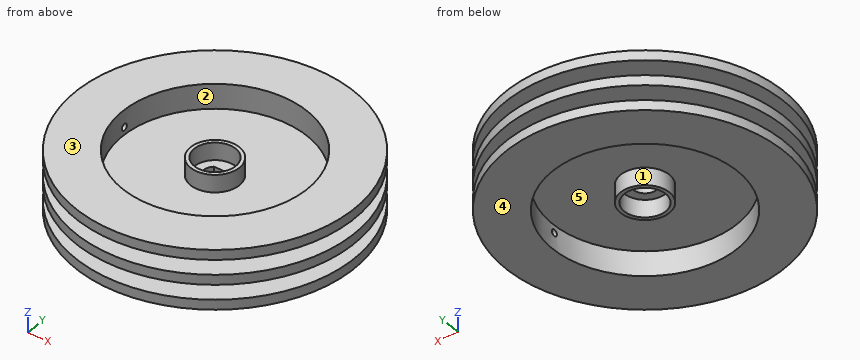
```python
from build123d import *

# Parameters (mm, degrees)
SKETCH1_R               = 23.9268
BOSS_EXTRUDE1_DEPTH     = 1.70942
SKETCH2_R               = 19.0119
BOSS_EXTRUDE2_DEPTH     = 2.54
SKETCH3_R               = 19.0119
BOSS_EXTRUDE3_DEPTH     = 2.54
SKETCH4_R               = 23.9268
BOSS_EXTRUDE4_DEPTH     = 1.70942
SKETCH5_R               = 23.9268
BOSS_EXTRUDE5_DEPTH     = 1.70942
SKETCH6_R               = 15.875
CUT_EXTRUDE1_DEPTH      = 4.24942
SKETCH7_R               = 15.875
CUT_EXTRUDE2_DEPTH      = 4.24942
SKETCH8_R               = 0.5715
CUT_EXTRUDE3_DEPTH      = 24.9268
CUT_EXTRUDE3_DEPTH_BACK = 24.9268
CUT_EXTRUDE4_DEPTH      = 6.9588401
SKETCH10_R              = 4.1975
SKETCH10_R_2            = 3.5625
BOSS_EXTRUDE7_DEPTH     = 3
SKETCH11_R              = 4.1975
SKETCH11_R_2            = 3.5625
BOSS_EXTRUDE8_DEPTH     = 3


with BuildPart() as part:
    # Sketch1 → Boss-Extrude1 (new body)
    with BuildSketch(Plane.XY):
        Circle(SKETCH1_R)
    extrude(amount=BOSS_EXTRUDE1_DEPTH)

    # Sketch2 → Boss-Extrude2 (add)
    with BuildSketch(Plane.XY.offset(1.70942)):
        Circle(SKETCH2_R)
    extrude(amount=BOSS_EXTRUDE2_DEPTH)

    # Sketch3 → Boss-Extrude3 (add)
    with BuildSketch(Plane(origin=(0, 0, 0), x_dir=(-1, 0, 0), z_dir=(0, 0, -1))):
        Circle(SKETCH3_R)
    extrude(amount=BOSS_EXTRUDE3_DEPTH)

    # Sketch4 → Boss-Extrude4 (add)
    with BuildSketch(Plane.XY.offset(4.24942)):
        Circle(SKETCH4_R)
    extrude(amount=BOSS_EXTRUDE4_DEPTH)

    # Sketch5 → Boss-Extrude5 (add)
    with BuildSketch(Plane(origin=(0, 0, -2.54), x_dir=(-1, 0, 0), z_dir=(0, 0, -1))):
        Circle(SKETCH5_R)
    extrude(amount=BOSS_EXTRUDE5_DEPTH)

    # Sketch6 → Cut-Extrude1 (cut)
    with BuildSketch(Plane.XY.offset(5.95884)):
        Circle(SKETCH6_R)
    extrude(amount=-CUT_EXTRUDE1_DEPTH, mode=Mode.SUBTRACT)

    # Sketch7 → Cut-Extrude2 (cut)
    with BuildSketch(Plane(origin=(0, 0, -4.24942), x_dir=(-1, 0, 0), z_dir=(0, 0, -1))):
        Circle(SKETCH7_R)
    extrude(amount=-CUT_EXTRUDE2_DEPTH, mode=Mode.SUBTRACT)

    # Sketch8 → Cut-Extrude3 (cut, two sides)
    with BuildSketch(Plane(origin=(0, 0, 0), x_dir=(0, 0, -1), z_dir=(1, 0, 0))) as cut_extrude3_sk:
        with Locations((-2.97942, 0)):
            Circle(SKETCH8_R)
        with Locations((1.27, 0)):
            Circle(SKETCH8_R)
    extrude(amount=CUT_EXTRUDE3_DEPTH, mode=Mode.SUBTRACT)
    extrude(cut_extrude3_sk.sketch, amount=-CUT_EXTRUDE3_DEPTH_BACK, mode=Mode.SUBTRACT)

    # Sketch9 → Cut-Extrude4 (cut, through all)
    with BuildSketch(Plane.XY.offset(1.70942)):
        with BuildLine():
            Line((-1.322875656, 1.5), (1.322875656, 1.5))
            ThreePointArc((1.322875656, 1.5), (0, -2), (-1.322875656, 1.5))
        make_face()
    extrude(amount=-CUT_EXTRUDE4_DEPTH, mode=Mode.SUBTRACT)

    # Sketch10 → Boss-Extrude7 (add)
    with BuildSketch(Plane.XY.offset(1.70942)):
        Circle(SKETCH10_R)
        Circle(SKETCH10_R_2, mode=Mode.SUBTRACT)
    extrude(amount=BOSS_EXTRUDE7_DEPTH)

    # Sketch11 → Boss-Extrude8 (add)
    with BuildSketch(Plane(origin=(0, 0, 0), x_dir=(-1, 0, 0), z_dir=(0, 0, -1))):
        Circle(SKETCH11_R)
        Circle(SKETCH11_R_2, mode=Mode.SUBTRACT)
    extrude(amount=BOSS_EXTRUDE8_DEPTH)


solid = part.part
```
Here's how the part is built. I have some questions about the finished solid (model axes, mm). Face numbers are marked on the shaded views. A direction names the side the tool comes from. Coordinates: 2 decimals unless noted, no trailing zeros. Order: outer loops, then holes, each group sorted by start corner. A loop starts at its lowest first (then second) coordinate and runs counter-clockwise, first axis right, second up. Notation, with made-up numbers: (25.5, 50.5) - (60.5, 50.5) arc R19 ccw to (60.5, 71.5) - close; hole circle Ø3 at (18, -39.5). An arc over 180 degrees is marked (long way). One line per question, with ' | ' between items. Start each with the question number.
1. If we section it at A-A (z = -1.27): Give the number of separate pieces and of enclosed holes in the cut face, and give its area (3 significant figures).
2. I'm going to push flat-ended pins straight in: pin 1 Ø6 at (y, z) = (17.5, -3) entering from -X; pin 2 Ø4.5 at (x, y) = (0, 0) entering from -Z; pin 3 Ø6 at (x, z) = (-2, 3) entering from -Y. Where does each tip first touch, or does it pass through?
3. If we section it at B-B (x = 17): Write out the boundary of the cut face in (y, z).
4. If we section it at D-D (x = -6): Write out the boundary of the cut face in (y, z).
5. Please list where these lines run through material, in increasing order: line 1 along Z through (x, y) = (21, 3.5); line 2 along Y through (x, z) = (0, -2.45) (1 decimal); line 3 along X through (y, z) = (2, 3). Write a range as [from, to].
6. Which directions (+Z, -Z, +X, -X, +Y, -Y) give clear straight access to the entire face, cutting with the end or side of a thin tool? Please do the marked faces 1, 2 and 3.
7. If we mould it in two halves opening along X, with no side actions, what happens to the marked faces 4 and 5? For each: released by +X, released by -X, zero draft, split by the parting line, or undercut.
8. If we section it at C-C (y = -17): Write out the boundary of the cut face in (x, z), and give its area (3 significant figures).
Model answer:
1) separate pieces: 3 | enclosed holes: 1 | area: 352 mm²
2) pin 1: stops at x = -19.03 | pin 2: stops at z = 0 | pin 3: stops at y = -23.93
3) outline: (-16.84, -4.25) - (16.84, -4.25) - (16.84, -2.54) - (8.51, -2.54) - (8.51, 0) - (16.84, 0) - (16.84, 1.71) - (8.51, 1.71) - (8.51, 4.25) - (16.84, 4.25) - (16.84, 5.96) - (-16.84, 5.96) - (-16.84, 4.25) - (-8.51, 4.25) - (-8.51, 1.71) - (-16.84, 1.71) - (-16.84, 0) - (-8.51, 0) - (-8.51, -2.54) - (-16.84, -2.54) - close; hole circle Ø1.14 at (0, -1.27); hole circle Ø1.14 at (0, 2.98)
4) outline: (-23.16, -4.25) - (-14.7, -4.25) - (-14.7, 0) - (14.7, 0) - (14.7, -4.25) - (23.16, -4.25) - (23.16, -2.54) - (18.04, -2.54) - (18.04, 0) - (23.16, 0) - (23.16, 1.71) - (18.04, 1.71) - (18.04, 4.25) - (23.16, 4.25) - (23.16, 5.96) - (14.7, 5.96) - (14.7, 1.71) - (-14.7, 1.71) - (-14.7, 5.96) - (-23.16, 5.96) - (-23.16, 4.25) - (-18.04, 4.25) - (-18.04, 1.71) - (-23.16, 1.71) - (-23.16, 0) - (-18.04, 0) - (-18.04, -2.54) - (-23.16, -2.54) - close
5) line 1: z = [-4.25, -2.54], [0, 1.71], [4.25, 5.96] | line 2: y = [-19, -15.9], [-4.2, -3.6], [3.6, 4.2], [15.9, 19] | line 3: x = [-18.91, -15.75], [-3.69, -2.95], [2.95, 3.69], [15.75, 18.91]
6) face 1: -Z | face 2: +Z | face 3: +Z, +X, -X, +Y, -Y
7) face 4: zero draft | face 5: undercut
8) outline: (-16.84, -4.25) - (16.84, -4.25) - (16.84, -2.54) - (8.51, -2.54) - (8.51, 0) - (16.84, 0) - (16.84, 1.71) - (8.51, 1.71) - (8.51, 4.25) - (16.84, 4.25) - (16.84, 5.96) - (-16.84, 5.96) - (-16.84, 4.25) - (-8.51, 4.25) - (-8.51, 1.71) - (-16.84, 1.71) - (-16.84, 0) - (-8.51, 0) - (-8.51, -2.54) - (-16.84, -2.54) - close | area: 259 mm²
